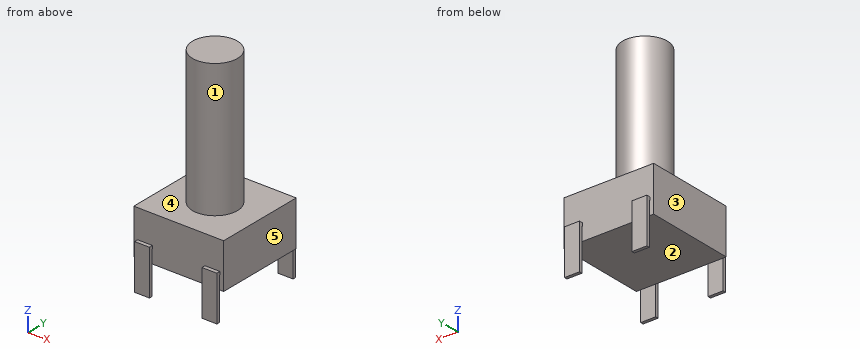
```python
from build123d import *

# Parameters (mm, degrees)
SKETCH_1_W               = 6
SKETCH_1_H               = 6
EXTRUDE_1_DEPTH          = 3
SKETCH_2_R               = 1.5
EXTRUDE_2_DEPTH          = 9
SKETCH_4_W               = 1
SKETCH_4_H               = 0.2
MIRROR_2_COPY_1_SKETCH_W = 1
MIRROR_2_COPY_1_SKETCH_H = 0.2


with BuildPart() as part:
    # 草图1 → 凸台-拉伸1 (new body)
    with BuildSketch(Plane.XY):
        Rectangle(SKETCH_1_W, SKETCH_1_H)
    extrude(amount=EXTRUDE_1_DEPTH)

    # 草图2 → 凸台-拉伸2 (add)
    with BuildSketch(Plane.XY.offset(3)):
        with Locations(Location((0, 0, 0), (0, 0, 180))):
            Circle(SKETCH_2_R)
    extrude(amount=EXTRUDE_2_DEPTH)

    # 扫描3: sweep along a path in 草图6
    with BuildLine(Plane(origin=(2.25, 0, 0), x_dir=(0, 0, -1), z_dir=(1, 0, 0))) as sweep_3_path:
        Line((-1.1, -3), (-1.1, -3.25))
        Line((-1.1, -3.25), (1.9, -3.25))
    # 草图4 → 扫描3 (sweep)
    with BuildSketch(Plane.XZ.offset(3)):
        with Locations((2.25, 1)):
            Rectangle(SKETCH_4_W, SKETCH_4_H)
    sweep_3 = sweep(path=sweep_3_path.line, transition=Transition.RIGHT)

    # 镜向1: 扫描3 across plane
    add(sweep_3.mirror(Plane(origin=(0, 0, 0), x_dir=(0, 0, 1), z_dir=(1, 0, 0))))

    # 镜向2: 扫描3 across plane
    add(sweep_3.mirror(Plane.ZX))

    # 镜向2 copy 1: sweep along a path in 镜向2 copy 1 path
    with BuildLine(Plane(origin=(-2.25, 0, 0), x_dir=(0, 0, -1), z_dir=(-1, 0, 0))) as mirror_2_copy_1_path:
        Line((-1.1, -3), (-1.1, -3.25))
        Line((-1.1, -3.25), (1.9, -3.25))
    # 镜向2 copy 1 sketch → 镜向2 copy 1 (sweep)
    with BuildSketch(Plane(origin=(0, 3, 0), x_dir=(-1, 0, 0), z_dir=(0, 1, 0))):
        with Locations((2.25, 1)):
            Rectangle(MIRROR_2_COPY_1_SKETCH_W, MIRROR_2_COPY_1_SKETCH_H)
    sweep(path=mirror_2_copy_1_path.line, transition=Transition.RIGHT)


solid = part.part
```
Part model, mm, in its own coordinate system. Face numbers are marked on the shaded views. A direction names the side the tool comes from. Round coordinates to 2 decimals unless told otherwise and drop trailing zeros. Write each loop counter-clockwise with the first axis right and the second up, starting at its lowest first coordinate (ties: lowest second). Pieces come first, ordered by that corner, then holes. Notation, with made-up numbers: M 21.5,-37 L 45.5,-37 A21 ccw 45.5,-30 Z; hole C 18,45.25 d6. An arc over 180 degrees is marked long. Answer as CSV lines item,"result". Start each with the question number.
1) Drill centre lines: L1, parallel to Z at x = 0.2, y = 1.75; L2, parallel to Z at x = 0.15, y = 1; L3, parallel to Y at x = -1.1, z = 2.5. Where is each one in solid material? Low to high.
2) Band-saw the part on B-B (x = 0). List the corners of the cut face in (y, z).
3) Band-saw the part on A-A (z = 0.25). List the corners of the cut face in (x, y).
4) Band-saw the part on D-D (z = 9.25). List the corners of the cut face in (x, y).
5) Which spindle directions (+Z, -Z, +X, -X, +Y, -Y) get a long thin tool onto all of the face, cutting with end or side? Do the marked faces 4 and 5. Say none if no direction does.
6) Mould opens along Y. For the marked faces 1, 2 and 3 say: +Y half, -Y half, draft (parallel to the pull), parting line (faces both ways), or undercut.
7) Drop flat-ended pins along their axis: pin 1 (2 mm diameter, centred on x = 0, z = 2, fed in from +Y); pin 2 (3 mm diameter, centred on x = 1.5, y = 0, fed in from -Z); pin 3 (1.5 mm diameter, centred on y = -0.5, z = 4.5, fed in from -X). Give the stop position or say it passes through.
Worked out:
1,L1,"0 to 3"
1,L2,"0 to 12"
1,L3,"-3 to 3"
2,outline,"M -3,0 L 3,0 L 3,3 L 1.5,3 L 1.5,12 L -1.5,12 L -1.5,3 L -3,3 Z"
3,outline,"M -3,-3 L 3,-3 L 3,3 L -3,3 Z; M -2.75,-3.25 L -1.75,-3.25 L -1.75,-3.05 L -2.75,-3.05 Z; M -2.75,3.05 L -1.75,3.05 L -1.75,3.25 L -2.75,3.25 Z; M 1.75,-3.25 L 2.75,-3.25 L 2.75,-3.05 L 1.75,-3.05 Z; M 1.75,3.05 L 2.75,3.05 L 2.75,3.25 L 1.75,3.25 Z"
4,outline,"C 0,0 d3"
5,face 4,"+Z"
5,face 5,"+Z, -Z, +X, +Y, -Y"
6,face 1,"parting line"
6,face 2,"undercut"
6,face 3,"draft"
7,pin 1,"y = 3"
7,pin 2,"z = 0"
7,pin 3,"x = -1.5"
